Model file for the job. Use its own axes, mm. A direction names the side the tool comes from. Coordinates: 2 decimals unless noted, no trailing zeros. Write each loop counter-clockwise with the first axis right and the second up, starting at its lowest first coordinate (ties: lowest second). Pieces come first, ordered by that corner, then holes.
Q1. Band-saw the part on D-D, the plane x = -33.5. Write the cut outline in (y, z), plus the area to 3 significant figures.
Q2. Pull direction Z, two halves, no side cores. Call faces 4 (the flat face through (-73, 3, 0)), 5 (the flat face through (15, 3, -27.45)), 6 (the cylindrical face through (-34.68, 2.96, -16.58)), 7 (the cylindrical face through (-23.196, 2.958, 38.289)): released by +Z, released by -Z, zero draft, split by the parting line, or undercut.
Q3. Pin check, flat tips, straight feed: P1, Ø3, axis at x = 18.605, z = 10, coming from the +Y side; P2, Ø0.9, axis at y = 3.5, z = -32.5, coming from the -X side; P3, Ø1.8, axis at x = -41.5, y = 2, coming from the +Z side; P4, Ø2, axis at x = -50.5, y = 1, coming from the -Z side. Stop position of each tip, or through.
Q4. Band-saw the part on C-C, the plane y = 1.75. State how many separate pieces and enclosed holes the cut face has, plus the area to 3 significant figures.
Q5. Band-saw the part on A-A, the plane z = 0. Write the cut outline in (x, y), plus the area to 3 significant figures.
Q6. Which spindle directions (+Z, -Z, +X, -X, +Y, -Y) get a long thin tool onto all of the face, cutting with end or side? Do faces 1 (the flat face through (-25, 3, -32)), 2 (the cylindrical face through (18.55, 2.96, 29.94)), 3 (the flat face through (-70, 3, 22)). Say none if no direction does.
Q7. Band-saw the part on B-B, the plane x = -49. Write the cut outline in (y, z).
Q8. Drill centre lines: probe 1 along Z at (x, y) = (-33.5, 3.1); probe 2 along X at (y, z) = (1.3, 15.5); probe 3 along X at (y, z) = (5, 29). Where is each one in solid material? Low to high.
from build123d import *

# Parameters (mm, degrees)
SKETCH_1_R          = 11.25
SKETCH_1_R_2        = 1.6
SKETCH_1_R_3        = 2.550000002
EXTRUDE_1_DEPTH     = 6
SKETCH_2_R          = 2.55
CUT_EXTRUDE_1_DEPTH = 7


with BuildPart() as part:
    # Эскиз1 → Бобышка-Вытянуть1 (new body)
    with BuildSketch(Plane(origin=(0, 0, 0), x_dir=(1, 0, 0), z_dir=(0, 1, 0))):
        with BuildLine():
            Line((-32, -24), (-68, -24))
            Line((-68, -24), (-73, -19))
            Line((-73, -19), (-73, 19))
            Line((-73, 19), (-68, 24))
            Line((-68, 24), (-32, 24))
            ThreePointArc((-32, 24), (-27.050252532, 26.050252532), (-25, 31))
            Line((-25, 31), (-25, 34))
            ThreePointArc((-25, 34), (-23.242640687, 38.242640687), (-19, 40))
            Line((-19, 40), (19, 40))
            ThreePointArc((19, 40), (23.242640687, 38.242640687), (25, 34))
            Line((25, 34), (25, -34))
            ThreePointArc((25, -34), (23.242640687, -38.242640687), (19, -40))
            Line((19, -40), (-19, -40))
            ThreePointArc((-19, -40), (-23.242640687, -38.242640687), (-25, -34))
            Line((-25, -34), (-25, -31))
            ThreePointArc((-25, -31), (-27.050252532, -26.050252532), (-32, -24))
        make_face()
        with Locations((-49, 0)):
            Circle(SKETCH_1_R, mode=Mode.SUBTRACT)
        with Locations((-64.5, 15.5)):
            Circle(SKETCH_1_R_2, mode=Mode.SUBTRACT)
        with Locations((-64.5, -15.5)):
            Circle(SKETCH_1_R_2, mode=Mode.SUBTRACT)
        with Locations((-33.5, 15.5)):
            Circle(SKETCH_1_R_2, mode=Mode.SUBTRACT)
        with Locations((-33.5, -15.5)):
            Circle(SKETCH_1_R_2, mode=Mode.SUBTRACT)
        with Locations((18.604999997, -10)):
            Circle(SKETCH_1_R_3, mode=Mode.SUBTRACT)
        with Locations((18.604999997, 10)):
            Circle(SKETCH_1_R_3, mode=Mode.SUBTRACT)
    extrude(amount=EXTRUDE_1_DEPTH)

    # Эскиз2 → Вырез-Вытянуть1 (cut, through all)
    with BuildSketch(Plane.XZ):
        with Locations((-17, -30)):
            Circle(SKETCH_2_R)
        with Locations((-17, 30)):
            Circle(SKETCH_2_R)
        with BuildLine():
            Line((16, -32.55), (14, -32.55))
            ThreePointArc((14, -32.55), (11.45, -30), (14, -27.45))
            Line((14, -27.45), (16, -27.45))
            ThreePointArc((16, -27.45), (18.55, -30), (16, -32.55))
        make_face()
        with BuildLine():
            Line((16, 32.55), (14, 32.55))
            ThreePointArc((14, 32.55), (11.45, 30), (14, 27.45))
            Line((14, 27.45), (16, 27.45))
            ThreePointArc((16, 27.45), (18.55, 30), (16, 32.55))
        make_face()
    extrude(amount=-CUT_EXTRUDE_1_DEPTH, mode=Mode.SUBTRACT)


solid = part.part
Answer sheet:
1. outline: (0, -24) - (6, -24) - (6, -17.1) - (0, -17.1) - close; (0, -13.9) - (6, -13.9) - (6, 13.9) - (0, 13.9) - close; (0, 17.1) - (6, 17.1) - (6, 24) - (0, 24) - close
1. area: 250 mm2
2. face 4: zero draft
2. face 5: undercut
2. face 6: undercut
2. face 7: released by +Z
3. P1: passes through
3. P2: stops at x = -25
3. P3: stops at z = 24
3. P4: stops at z = -24
4. separate pieces: 1
4. enclosed holes: 11
4. area: 5,700 mm2
5. outline: (-73, 0) - (-60.25, 0) - (-60.25, 6) - (-73, 6) - close; (-37.75, 0) - (25, 0) - (25, 6) - (-37.75, 6) - close
5. area: 453 mm2
6. face 1: -Z, -X, +Y, -Y
6. face 2: +Y, -Y
6. face 3: +Z, -X, +Y, -Y
7. outline: (0, -24) - (6, -24) - (6, -11.25) - (0, -11.25) - close; (0, 11.25) - (6, 11.25) - (6, 24) - (0, 24) - close
8. probe 1: z = -24 to -17.1, -13.9 to 13.9, 17.1 to 24
8. probe 2: x = -73 to -66.1, -62.9 to -35.1, -31.9 to 25
8. probe 3: x = -25.29 to -19.35, -14.65 to 11.65, 18.35 to 25
